```python
from build123d import *

# Parameters (mm, degrees)
SKETCH1_R               = 42.5
BOSS_EXTRUDE1_DEPTH     = 10
SKETCH2_R               = 5
BOSS_EXTRUDE2_DEPTH     = 7
SKETCH3_R               = 2
BOSS_EXTRUDE3_DEPTH     = 5
CUT_EXTRUDE1_DEPTH      = 63.461988577
CUT_EXTRUDE1_DEPTH_BACK = 63.461988577
SKETCH3_4_R             = 2


with BuildPart() as part:
    # Sketch1 → Boss-Extrude1 (new body)
    with BuildSketch(Plane(origin=(0, 0, 0), x_dir=(1, 0, 0), z_dir=(0, 1, 0))):
        with Locations(Location((0, 0, 0), (0, 0, 270))):
            Circle(SKETCH1_R)
    extrude(amount=BOSS_EXTRUDE1_DEPTH)

    # Sketch2 → Boss-Extrude2 (add)
    with BuildSketch(Plane.XZ):
        with Locations(Location((-21.003335433, 21.421015399, 0), (0, 0, 90))):
            Circle(SKETCH2_R)
        with Locations(Location((21.421015399, 21.003335433, 0), (0, 0, 90))):
            Circle(SKETCH2_R)
        with Locations(Location((21.003335433, -21.421015399, 0), (0, 0, 90))):
            Circle(SKETCH2_R)
        with Locations(Location((-21.421015399, -21.003335433, 0), (0, 0, 90))):
            Circle(SKETCH2_R)
    extrude(amount=BOSS_EXTRUDE2_DEPTH)

    # Sketch3 → Boss-Extrude3 (add)
    with BuildSketch(Plane(origin=(0, 10, 0), x_dir=(1, 0, 0), z_dir=(0, 1, 0))):
        with BuildLine():
            ThreePointArc((7.410610084, 9.984822024), (12.938182194, 0.241771609), (7.815144583, -9.719933589))
            ThreePointArc((7.815144583, -9.719933589), (14.183962111, -19.037364236), (25.178047354, -16.486591759))
            add(Edge.make_bspline(
                [(29, -6.35), (28.699050384, -11.600454078), (25.178047354, -16.486591759)],
                knots=[0.67268265, 0.67268265, 0.67268265, 1, 1, 1], degree=2))
            add(Edge.make_bspline(
                [(29, 6.35), (30.042272144, 0), (29, -6.35)],
                knots=[0, 0, 0, 1, 1, 1], degree=2))
            add(Edge.make_bspline(
                [(26.688052402, 13.325870914), (27.746594537, 11.107404767), (28.624649084, 8.772780294), (29, 6.35)],
                knots=[0.050650552, 0.050650552, 0.050650552, 0.050650552, 0.277553495, 0.277553495, 0.277553495, 0.277553495], degree=3))
            add(Edge.make_bspline(
                [(25.95577439, 14.793850517), (26.206471304, 14.310519768), (26.451758672, 13.821089407), (26.688052402, 13.325870914)],
                knots=[0, 0, 0, 0, 0.050650552, 0.050650552, 0.050650552, 0.050650552], degree=3))
            ThreePointArc((25.95577439, 14.793850517), (14.893502945, 19.290955178), (7.410610084, 9.984822024))
        make_face()
        with Locations(Location((24.5, 0, 0), (0, 0, 270))):
            Circle(SKETCH3_R, mode=Mode.SUBTRACT)
        with Locations(Location((17.25, 0, 0), (0, 0, 270))):
            Circle(SKETCH3_R, mode=Mode.SUBTRACT)
    extrude(amount=BOSS_EXTRUDE3_DEPTH)

    # Sketch3_4 → Cut-Extrude1 (cut, two sides: drawn at the far end of the back side and taken through both)
    with BuildSketch(Plane(origin=(0, 10, 0), x_dir=(1, 0, 0), z_dir=(0, 1, 0)).offset(-CUT_EXTRUDE1_DEPTH_BACK)):
        with Locations(Location((24.5, 0, 0), (0, 0, 270))):
            Circle(SKETCH3_4_R)
        with Locations(Location((17.25, 0, 0), (0, 0, 270))):
            Circle(SKETCH3_4_R)
    extrude(amount=CUT_EXTRUDE1_DEPTH + CUT_EXTRUDE1_DEPTH_BACK, mode=Mode.SUBTRACT)


solid = part.part
```
Verification items for the finished model (mm, model axes). A direction names the side the tool comes from. Round coordinates to 2 decimals unless told otherwise and drop trailing zeros. Order: outer loops, then holes, each group sorted by start corner. A loop starts at its lowest first (then second) coordinate and runs counter-clockwise, first axis right, second up. Notation, with made-up numbers: (58.5, 69) -> (96.5, 69) arc R20 cw to (96.5, 102) -> close; hole circle Ø7 at (-18.5, -19). An arc over 180 degrees is marked (long way). Put each result on its own line as item: value. Start each with the question number.
(1) Section check C-C (x = 0). Enter the section's corners in (y, z).
(2) Section check A-A (y = 6.75). Enter the section's corners in (x, z), then the cut area to 3 significant figures.
(3) Section check D-D (z = 0). State how many separate pieces and enclosed holes the cut face has, then the cut area to 3 significant figures.
(4) Depth check by flat-ended pin: pin 1 Ø4.5 at (x, z) = (17.25, 0) entering from -Y; pin 2 Ø5 at (x, y) = (-3, 10.5) entering from +Z; pin 3 Ø8 at (x, y) = (-13, 12.5) entering from -Z. Enter the tip coordinate at first touch or a pass-through.
(5) Tool access check on faces 1 (the face through (14.028, 12.465, 18.975)), 2 (the face through (12.934, 12.465, -0.405)), 3 (the face through (15.067, 12.465, -19.334)), 4 (the face through (16.046, -3.451, -22.072)). Record the directions out of +Z, -Z, +X, -X, +Y, -Y that give a thin tool (end or side, any length) a straight path to the whole face; none if there is none.
(6) Section check B-B (z = 34). Enter the section's corners in (x, y).
(7) Material ranges on line 1 along X through (y, z) = (8.75, 0); line 2 along X through (y, z) = (10.5, 0); line 3 along Z through (x, y) = (24.5, 11.25), recorded low to high.
(8) Draft check along X on faces 5 (the face through (-25.861, 4.93, -33.727)), 6 (the face through (1, 10, -1)), 7 (the face through (19.233, 7.395, -0.26)). Enter one of: +X half, -X half, draft (parallel to the pull), parting line (faces both ways), or undercut.
Completed:
1. outline: (0, -42.5) -> (10, -42.5) -> (10, 42.5) -> (0, 42.5) -> close
2. outline: circle Ø85 at (0, 0); hole circle Ø4 at (17.25, 0); hole circle Ø4 at (24.5, 0)
2. area: 5,650 mm2
3. separate pieces: 3
3. enclosed holes: 0
3. area: 813 mm2
4. pin 1: stops at y = 0
4. pin 2: stops at z = 42.5
4. pin 3: stops at z = -41.34
5. face 1: +Z, +Y
5. face 2: -X, +Y
5. face 3: -Z, +Y
5. face 4: -Y
6. outline: (-25.5, 0) -> (25.5, 0) -> (25.5, 10) -> (-25.5, 10) -> close
7. line 1: x = -42.5 to 15.25, 19.25 to 22.5, 26.5 to 42.5
7. line 2: x = 12.94 to 15.25, 19.25 to 22.5, 26.5 to 29.52
7. line 3: z = -16.66 to -2, 2 to 17.16
8. face 5: parting line
8. face 6: draft
8. face 7: undercut
